Can you work these out from the drawing? Everything is in mm from the part's minimum corner. A direction names the side the tool comes from. Round coordinates to 2 decimals unless told otherwise and drop trailing zeros. Order: outer loops, then holes, each group sorted by start corner. A loop starts at its lowest first (then second) coordinate and runs counter-clockwise, first axis right, second up. Notation, with made-up numbers: M -28.5,32 L 11.5,32 A16 ccw 11.5,50 Z; hole C -39.5,19 d1. An arc over 180 degrees is marked long. Write each question's results on one line, items separated by ' | '. Start each with the question number.
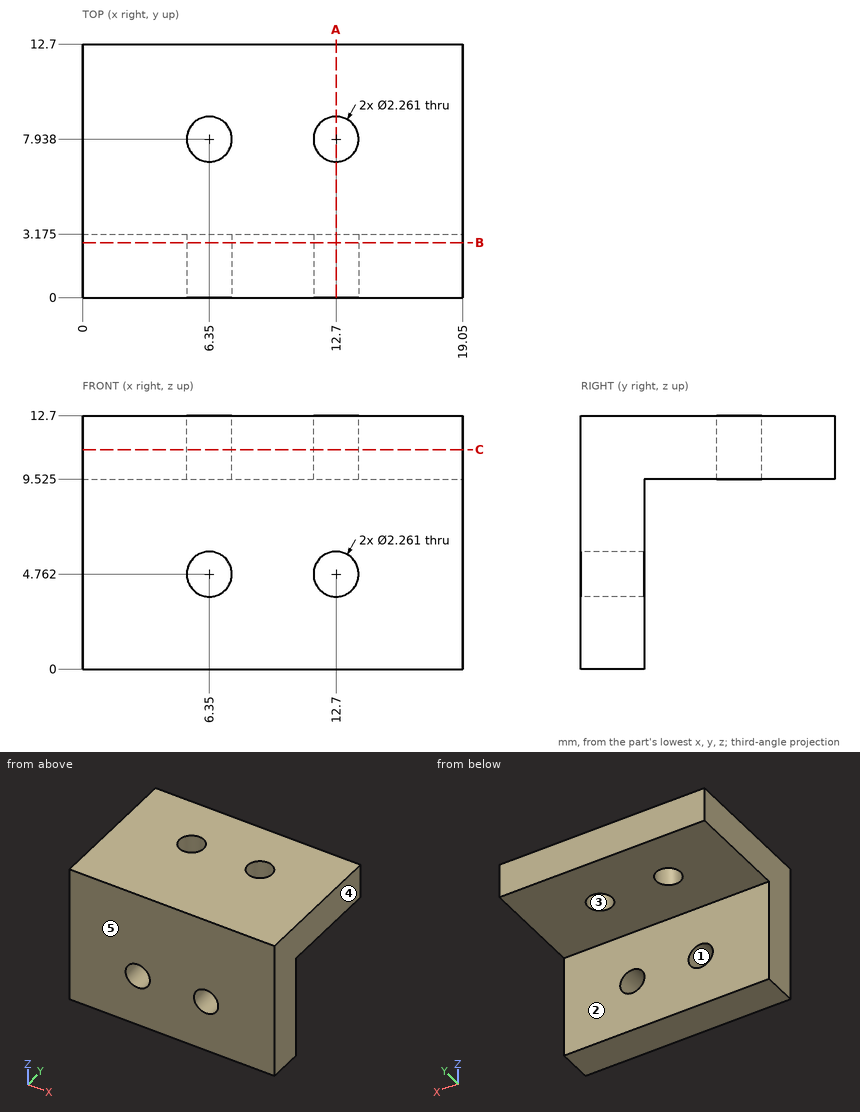
(1) I want a section at A-A on x = 12.7. Write out the boundary of the cut face in (y, z) (1 decimal).
(2) If we mould it in two halves opening along X, with no side actions, what happens to the marked faces 3, 4 and 5? For each: pulls with the +X half, pulls with the -X half, needs draft (parallel to the pull), parting line crosses it, or undercut.
(3) Please list where these lines run through material, in increasing order: line 1 (Z direction, x = 12.7, y = 2.25); line 2 (Y direction, x = 12.7, z = 11.3); line 3 (Z direction, x = 16.5, y = 8.75) (1 decimal).
(4) I want a section at B-B on y = 2.75. Write out the boundary of the cut face in (x, z).
(5) I want a section at C-C on z = 11. Write out the boundary of the cut face in (x, y), and give its area (3 significant figures).
(6) I'm going to push flat-ended pins straight in: pin 1 Ø5 at (x, y) = (8, 10.5) entering from -Z (1 decimal); pin 2 Ø6 at (x, y) = (5.5, 7.5) entering from +Z; pin 3 Ø7.5 at (x, z) = (11, 5.5) entering from +Y (1 decimal). Where does each tip first touch, or does it pass through?
(7) On a 3-axis mill with a long thin cutter (end or side, diameter ignored), from which of +Z, -Z, +X, -X, +Y, -Y can I reach the whole of each face in a straight line? I mean the marked faces 1 and 2. Say none if no direction works.
Solutions:
1) outline: M 0,0 L 3.2,0 L 3.2,3.6 L 0,3.6 Z; M 0,5.9 L 3.2,5.9 L 3.2,9.5 L 6.8,9.5 L 6.8,12.7 L 0,12.7 Z; M 9.1,9.5 L 12.7,9.5 L 12.7,12.7 L 9.1,12.7 Z
2) face 3: undercut | face 4: pulls with the +X half | face 5: needs draft
3) line 1: 0 to 3.63, 5.89 to 12.7 | line 2: 0 to 6.81, 9.07 to 12.7 | line 3: 9.5 to 12.7
4) outline: M 0,0 L 19.05,0 L 19.05,12.7 L 0,12.7 Z; hole C 6.35,4.76 d2.26; hole C 12.7,4.76 d2.26
5) outline: M 0,0 L 19.05,0 L 19.05,12.7 L 0,12.7 Z; hole C 6.35,7.94 d2.26; hole C 12.7,7.94 d2.26 | area: 234 mm^2
6) pin 1: z = 9.5 | pin 2: z = 12.7 | pin 3: y = 3.2
7) face 1: +Y, -Y | face 2: -Z, +X, -X, +Y
